Check sheet for the modelled part. Datum: model origin and axes. Units: mm. Face numbers are marked on the shaded views. A direction names the side the tool comes from. Give positions to 0.01 mm unless a question says otherwise; leave off trailing zeros. Loops run counter-clockwise (first coordinate to the right, second up) from the corner with the lowest first, then second, coordinate; pieces in that order, holes last. Notation, with made-up numbers: (-28.5, -27) -> (5.5, -27) arc R30 cw to (5.5, -1) -> close; hole circle Ø4 at (37, 57). An arc over 180 degrees is marked (long way). Answer as CSV lines item,"result". Start each with the question number.
(1) Section check D-D on z = 46. Enter the section's corners in (x, y).
(2) Section check C-C on x = 110.5. Enter the section's corners in (y, z).
(3) Gauge pin test, flat ends, axial feed: pin 1 Ø1 at (x, y) = (62, -43) entering from -Z; pin 2 Ø11.5 at (x, y) = (136, -52) entering from +Z; pin 3 Ø8 at (x, z) = (116.5, 59) entering from -Y. Record the tip position at first contact, or that the pin passes through.
(4) Access from +Z, -Z, +X, -X, +Y, -Y to the whole of each face (thin tool, end or side, straight path). Record for the marked faces 1 and 2.
(5) Material ranges on line 1 (Z direction, x = 50.8, y = -50) (3 decimals); line 2 (Y direction, x = 170, z = 66.5); line 3 (Z direction, x = 140, y = -49), recorded low to high. Write a range as from..to.
(6) Section check B-B on x = 50.8. Enter the section's corners in (y, z) (3 decimals).
(7) Release check for a two-part mould opening along Y. For the marked faces 3, 4 and 5 record: pulls with the +Y half, pulls with the -Y half, needs draft (parallel to the pull), parting line crosses it, or undercut.
(8) Section check A-A on y = -46. Enter the section's corners in (x, z) (3 decimals).
from build123d import *

# Parameters (mm, degrees)
F0_W     = 203.2
F0_H     = 76.2
F1_DEPTH = 76.2
F2_W     = 101.6
F2_H     = 38.1
F3_DEPTH = 38.1
F4_SIZE  = 5.08
F6_D     = 6.35


with BuildPart() as f1:
    # F0 (on Front) → F1 (new body)
    with BuildSketch(Plane.XZ):
        with Locations((101.6, 38.1)):
            Rectangle(F0_W, F0_H)
    extrude(amount=F1_DEPTH)

    # F2 (on face) → F3 (cut)
    with BuildSketch(Plane.XY.offset(76.2)):
        with Locations((152.4, -57.15)):
            Rectangle(F2_W, F2_H)
    extrude(amount=-F3_DEPTH, mode=Mode.SUBTRACT)

    # F4
    f4_edges = [f1.edges().sort_by_distance(p)[0] for p in [
        (50.8, -76.2, 76.2),
        (101.6, 0, 76.2),
        (0, -38.1, 76.2),
        (101.6, -57.15, 76.2),
        (152.4, -38.1, 76.2),
        (203.2, -19.05, 76.2),
    ]]
    chamfer(f4_edges, length=F4_SIZE)

    # F6 (through all)
    with Locations(Plane.XZ.offset(76.2)):
        with Locations((50.8, 38.1)):
            Hole(F6_D / 2)


solid = f1.part
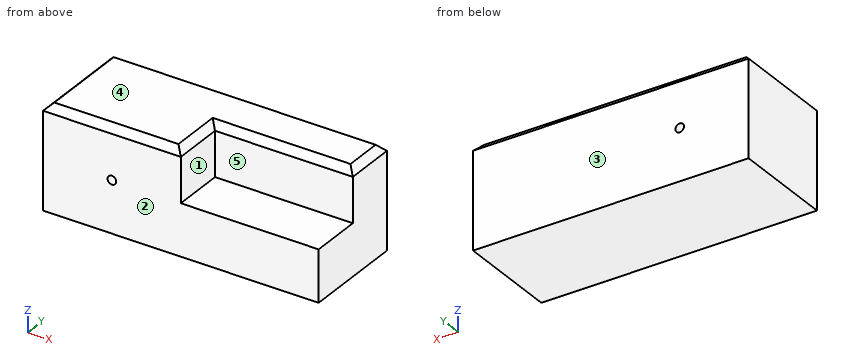
Working result:
1,outline,"(0, -76.2) -> (101.6, -76.2) -> (101.6, -38.1) -> (203.2, -38.1) -> (203.2, 0) -> (0, 0) -> close"
2,outline,"(-76.2, 0) -> (0, 0) -> (0, 71.12) -> (-5.08, 76.2) -> (-33.02, 76.2) -> (-38.1, 71.12) -> (-38.1, 38.1) -> (-76.2, 38.1) -> close"
3,pin 1,"stops at z = 0"
3,pin 2,"stops at z = 38.1"
3,pin 3,"stops at y = -38.1"
4,face 1,"+Z, +X, -Y"
4,face 2,"+Z, -Z, +X, -X, -Y"
5,line 1,"z = 0..34.925, 41.275..76.2"
5,line 2,"y = -38.1..0"
5,line 3,"z = 0..38.1"
6,outline,"(-76.2, 0) -> (0, 0) -> (0, 34.925) -> (-76.2, 34.925) -> close; (-76.2, 41.275) -> (0, 41.275) -> (0, 71.12) -> (-5.08, 76.2) -> (-71.12, 76.2) -> (-76.2, 71.12) -> close"
7,face 3,"pulls with the +Y half"
7,face 4,"needs draft"
7,face 5,"pulls with the -Y half"
8,outline,"(0, 0) -> (203.2, 0) -> (203.2, 38.1) -> (101.6, 38.1) -> (101.6, 71.12) -> (96.52, 76.2) -> (5.08, 76.2) -> (0, 71.12) -> close; hole circle Ø6.35 at (50.8, 38.1)"
